Drawing for the job (mm, zero at the part's lowest x, y, z). Give positions to 0.01 mm unless a question says otherwise; leave off trailing zeros. Write each loop counter-clockwise with the first axis right and the second up, starting at its lowest first coordinate (ties: lowest second). Pieces come first, ordered by that corner, then holes. Notation, with made-up numbers: M 55.5,38 L 92.5,38 A18 cw 92.5,58 Z; hole C 70,-8.75 d8. An arc over 180 degrees is marked long. Use CSV: the item, a comma, the result in double quotes. Start each with the question number.
1. Mould opens along X. For the marked faces 1, 2 and 3 say: pulls with the +X half, pulls with the -X half, needs draft (parallel to the pull), parting line crosses it, or undercut.
2. Band-saw the part on C-C, the plane y = 0.5. List the corners of the cut face in (x, z), then the cut area to 3 significant figures.
3. Drop flat-ended pins along their axis: pin 1 Ø4 at (y, z) = (3.5, 9) entering from -X; pin 2 Ø1.5 at (x, z) = (7, 12.5) entering from +Y; pin 3 Ø9.5 at (x, z) = (13.5, 13) entering from -Y; pin 4 Ø4 at (y, z) = (1.5, 9.5) entering from +X. Give the stop position or say it passes through.
4. Band-saw the part on B-B, the plane x = 15. List the corners of the cut face in (y, z), then the cut area to 3 significant figures.
5. Drill centre lines: line 1 along Z through (x, y) = (15, 6.8); line 2 along Z through (x, y) = (15, 4.65); line 3 along X through (y, z) = (3, 10.75). Where is each one in solid material? Low to high. Write a range as from..to.
6. Band-saw the part on D-D, the plane y = 5.25. List the corners of the cut face in (x, z).
7. Band-saw the part on A-A, the plane z = 15. List the corners of the cut face in (x, y).
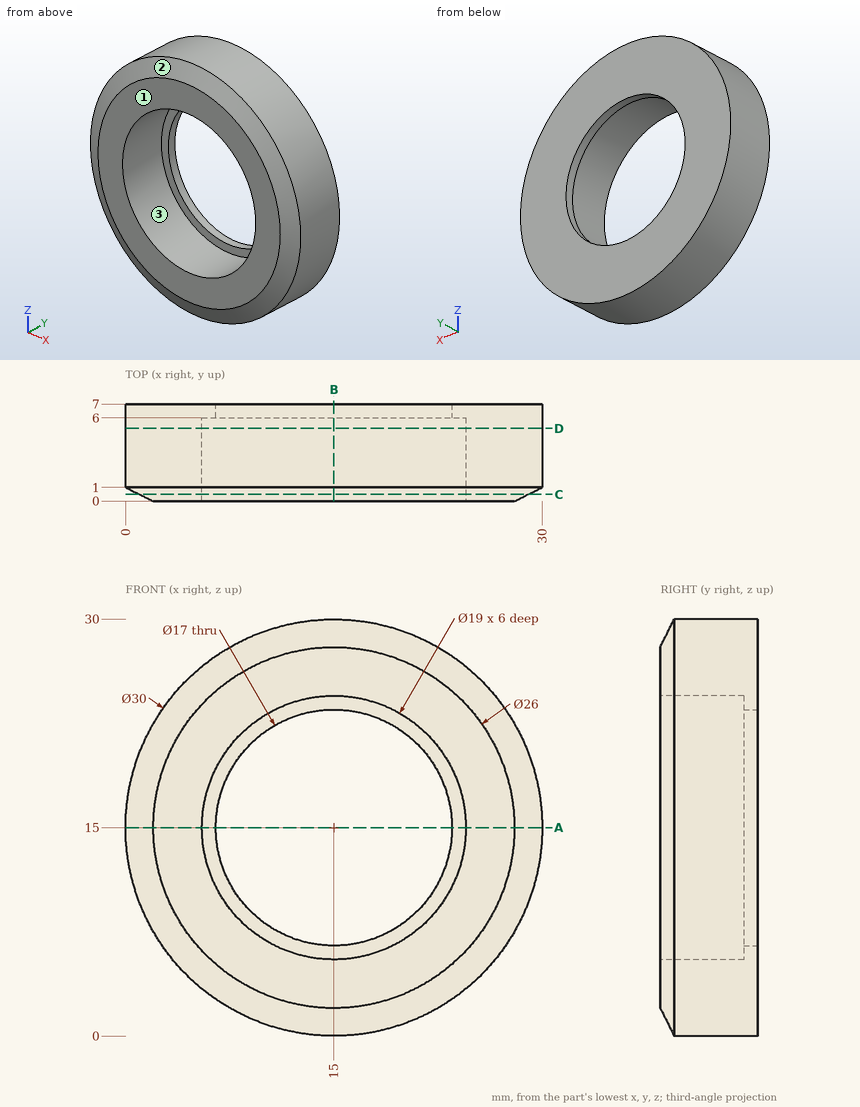
Output:
1,face 1,"needs draft"
1,face 2,"parting line crosses it"
1,face 3,"undercut"
2,outline,"C 15,15 d28; hole C 15,15 d19"
2,area,"332 mm²"
3,pin 1,"stops at x = 0.54"
3,pin 2,"stops at y = 7"
3,pin 3,"passes through"
3,pin 4,"stops at x = 29.59"
4,outline,"M 0,2 L 1,0 L 7,0 L 7,6.5 L 6,6.5 L 6,5.5 L 0,5.5 Z; M 0,24.5 L 6,24.5 L 6,23.5 L 7,23.5 L 7,30 L 1,30 L 0,28 Z"
4,area,"77.0 mm²"
5,line 1,"z = 0..6.5, 23.5..30"
5,line 2,"z = 0..5.5, 24.5..30"
5,line 3,"x = 0.61..6.5, 23.5..29.39"
6,outline,"C 15,15 d30; hole C 15,15 d19"
7,outline,"M 0,1 L 2,0 L 5.5,0 L 5.5,6 L 6.5,6 L 6.5,7 L 0,7 Z; M 23.5,6 L 24.5,6 L 24.5,0 L 28,0 L 30,1 L 30,7 L 23.5,7 Z"
